```python
from build123d import *

# Parameters (mm, degrees)
BOSS_EXTRUDE1_DEPTH = 10


with BuildPart() as part:
    # Sketch1 → Boss-Extrude1 (new, symmetric)
    with BuildSketch(Plane(origin=(0, 0, 0), x_dir=(1, 0, 0), z_dir=(0, 1, 0))):
        Polygon((15.294228634, 0.5), (7.5, 5), (7.5, 14), (-7.5, 14), (-7.5, 5), (-15.294228634, 0.5), (-7.794228634, -12.490381057), (0, -7.990381057), (7.794228634, -12.490381057), align=None)
    extrude(amount=BOSS_EXTRUDE1_DEPTH, both=True)


solid = part.part
```
CAD build for the part. Positions are in the model's coordinates, mm. A direction names the side the tool comes from. Round coordinates to 2 decimals unless told otherwise and drop trailing zeros. Write each loop counter-clockwise with the first axis right and the second up, starting at its lowest first coordinate (ties: lowest second). Pieces come first, ordered by that corner, then holes. Notation, with made-up numbers: (56, 52.5) -> (89, 52.5) arc R31 ccw to (89, 79.5) -> close; hole circle Ø2 at (82, 53.25). An arc over 180 degrees is marked (long way). Answer in a Markdown table with one row per item. Add a question column.
Item 1: Saw through at A-A, the plane y = 1.5. Write the cut outline in (x, z).
Item 2: Drop flat-ended pins along their axis: pin 1 Ø6 at (x, y) = (-11, 7.5) entering from +Z; pin 2 Ø2.5 at (y, z) = (-2.5, -10.5) entering from -X; pin 3 Ø2 at (x, y) = (-11, -8) entering from -Z; pin 4 Ø1.5 at (x, z) = (-10.5, -5) entering from -Y. Give the stop position or say it passes through.
Item 3: Drill centre lines: line 1 (X direction, y = -6.5, z = -6.75); line 2 (X direction, y = -3.25, z = 9.25); line 3 (X direction, y = -9, z = 10). Where is each one in solid material? Low to high. Write a range as from..to.
Item 4: Saw through at C-C, the plane x = 9. Write the cut outline in (y, z), then the cut area to 3 significant figures.
Item 5: Mould opens along X. For faces 1 (the face through (3.843, 0.14, 10.209)), 2 (the face through (11.49, 0.14, 6.09)), 3 (the face through (0, -10, -1)) say: pulls with the +X half, pulls with the -X half, needs draft (parallel to the pull), parting line crosses it, or undercut.
Item 6: Which spindle directions (+Z, -Z, +X, -X, +Y, -Y) get a long thin tool onto all of the face, cutting with end or side? Do faces 4 (the face through (-7.5, 0, -10)), 5 (the face through (0, 0, -14)), 6 (the face through (-4, 0.1, 10.3)), 7 (the face through (7.5, 0, -9)). Say none if no direction does.
Item 7: Saw through at B-B, the plane z = -7.25. Write the cut outline in (x, y).
Findings below:
| question | item | result |
|---|---|---|
| 1 | outline | (-15.29, -0.5) -> (-7.5, -5) -> (-7.5, -14) -> (7.5, -14) -> (7.5, -5) -> (15.29, -0.5) -> (7.79, 12.49) -> (0, 7.99) -> (-7.79, 12.49) -> close |
| 2 | pin 1 | stops at z = 12.13 |
| 2 | pin 2 | stops at x = -7.5 |
| 2 | pin 3 | stops at z = -3.56 |
| 2 | pin 4 | passes through |
| 3 | line 1 | x = -7.5..7.5 |
| 3 | line 2 | x = -9.67..-2.18, 2.18..9.67 |
| 3 | line 3 | x = -9.23..-3.48, 3.48..9.23 |
| 4 | outline | (-10, -4.13) -> (10, -4.13) -> (10, 10.4) -> (-10, 10.4) -> close |
| 4 | area | 291 mm^2 |
| 5 | face 1 | undercut |
| 5 | face 2 | pulls with the +X half |
| 5 | face 3 | needs draft |
| 6 | face 4 | -Z, -X, +Y, -Y |
| 6 | face 5 | -Z, +X, -X, +Y, -Y |
| 6 | face 6 | +Z, +Y, -Y |
| 6 | face 7 | -Z, +X, +Y, -Y |
| 7 | outline | (-7.5, -10) -> (7.5, -10) -> (7.5, 10) -> (-7.5, 10) -> close |
